Here's how the part is built. I have some questions about the finished solid (model axes, mm). Face numbers are marked on the shaded views. A direction names the side the tool comes from. Give positions to 0.01 mm unless a question says otherwise; leave off trailing zeros. Loops run counter-clockwise (first coordinate to the right, second up) from the corner with the lowest first, then second, coordinate; pieces in that order, holes last.
Q1. Suppose I cut it at D-D (x = 12). List the corners of the cut face in (y, z) for me, and give its area (3 significant figures).
Q2. Suppose I cut it at C-C (z = 14.5). List the corners of the cut face in (x, y) for me.
Q3. I'm going to push flat-ended pins straight in: P1, Ø1.6, axis at x = 13, z = 0.5, coming from the -Y side; P2, Ø2, axis at x = 12, z = 25.5, coming from the +Y side; P3, Ø1, axis at x = -14, z = 1.5, coming from the -Y side. Where does each tip first touch, or does it pass through?
Q4. For the marked faces 1 and 2, which set-ups out of +Z, -Z, +X, -X, +Y, -Y let a thin tool reach every point of the face, with its end or its side?
Q5. I need wall thicknesses on probe 1 along Z at (x, y) = (2, 24.25); probe 2 along Y at (x, z) = (14.5, 7.5); probe 3 along X at (y, z) = (-0.5, 25). Which ranges of each line are inside material? Lowest first, please.
Q6. Suppose I cut it at A-A (x = 0). List the corners of the cut face in (y, z) for me.
Q7. Suppose I cut it at B-B (y = 16.5). List the corners of the cut face in (x, z) for me.
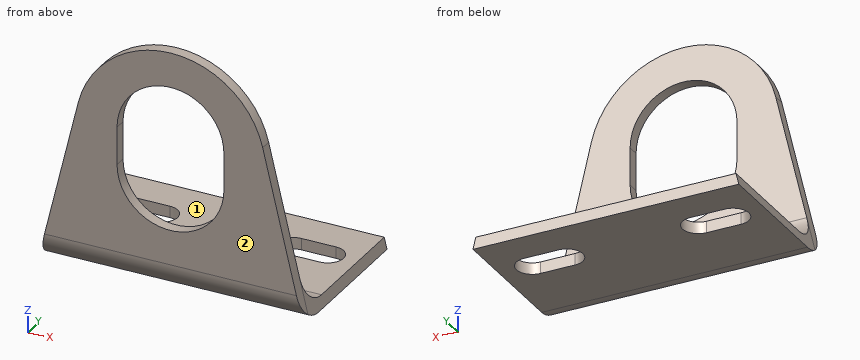
```python
from build123d import *

# Parameters (mm, degrees)
F1_DEPTH = 2
F3_DEPTH = 26
F4_R     = 5
F6_DEPTH = 2.001


with BuildPart() as f1:
    # F0 (on Front) → F1 (new body)
    with BuildSketch(Plane.XZ):
        with BuildLine():
            Line((-15.958655, 29.411045), (-23, 0))
            Line((-23, 0), (23, 0))
            Line((23, 0), (15.958655, 29.411045))
            ThreePointArc((15.958655, 29.411045), (0, 42), (-15.958655, 29.411045))
        make_face()
        with BuildLine():
            Line((-9.25, 20.25), (-9.25, 26.75))
            ThreePointArc((-9.25, 26.75), (0, 36), (9.25, 26.75))
            Line((9.25, 26.75), (9.25, 20.25))
            ThreePointArc((9.25, 20.25), (0, 11), (-9.25, 20.25))
        make_face(mode=Mode.SUBTRACT)
    extrude(amount=F1_DEPTH)

    # F2 (on face) → F3 (join)
    with BuildSketch(Plane(origin=(0, 0, 0), x_dir=(-1, 0, 0), z_dir=(0, 1, 0))):
        Polygon((22.521177, 2), (-22.521177, 2), (-23, 0), (23, 0), align=None)
    extrude(amount=F3_DEPTH)

    # F4
    f4_edges = [f1.edges().sort_by_distance(p)[0] for p in [
        (0, -2, 0),
        (0, 0, 2),
    ]]
    fillet(f4_edges, radius=F4_R)

    # F5 (on face) → F6 (cut, through all)
    with BuildSketch(Plane.XY.offset(2)):
        with BuildLine():
            Line((17.371177, 19.8), (11.371177, 19.8))
            ThreePointArc((11.371177, 19.8), (8.621177, 17.05), (11.371177, 14.3))
            Line((11.371177, 14.3), (17.371177, 14.3))
            ThreePointArc((17.371177, 14.3), (20.121177, 17.05), (17.371177, 19.8))
        make_face()
        with BuildLine():
            Line((-17.371177, 14.3), (-11.371177, 14.3))
            ThreePointArc((-11.371177, 14.3), (-8.621177, 17.05), (-11.371177, 19.8))
            Line((-11.371177, 19.8), (-17.371177, 19.8))
            ThreePointArc((-17.371177, 19.8), (-20.121177, 17.05), (-17.371177, 14.3))
        make_face()
    extrude(amount=-F6_DEPTH, mode=Mode.SUBTRACT)


solid = f1.part
```
Solutions:
1. outline: (-2, 5) arc R5 ccw to (3, 0) - (14.3, 0) - (14.3, 2) - (5, 2) arc R5 cw to (0, 7) - (0, 36.78) - (-2, 36.78) - close; (19.8, 0) - (26, 0) - (26, 2) - (19.8, 2) - close
1. area: 115 mm2
2. outline: (-19.53, -2) - (-7.25, -2) - (-7.25, 0) - (-19.53, 0) - close; (7.25, -2) - (19.53, -2) - (19.53, 0) - (7.25, 0) - close
3. P1: stops at y = -0.36
3. P2: stops at y = 0
3. P3: stops at y = -1
4. face 1: +Z, +X, -X, +Y
4. face 2: +Z, -Z, +X, -X, -Y
5. probe 1: z = 0 to 2
5. probe 2: y = -2 to 0
5. probe 3: x = -17.01 to -9.25, 9.25 to 17.01
6. outline: (-2, 5) arc R5 ccw to (3, 0) - (26, 0) - (26, 2) - (5, 2) arc R5 cw to (0, 7) - (0, 11) - (-2, 11) - close; (-2, 36) - (0, 36) - (0, 42) - (-2, 42) - close
7. outline: (-23, 0) - (-20.07, 0) - (-20.07, 2) - (-22.52, 2) - close; (-8.68, 0) - (8.68, 0) - (8.68, 2) - (-8.68, 2) - close; (20.07, 0) - (23, 0) - (22.52, 2) - (20.07, 2) - close
